Source: CAD feature listing. Evaluate the final solid. Frame: model axes, mm. A direction names the side the tool comes from. Give positions to 0.01 mm unless a question says otherwise; leave off trailing zeros. Order: outer loops, then holes, each group sorted by start corner. A loop starts at its lowest first (then second) coordinate and runs counter-clockwise, first axis right, second up.
from build123d import *

# Parameters (mm, degrees)
SKETCH_2_OUTSIDE_W  = 42.684
SKETCH_2_OUTSIDE_H  = 42.684
CUT_EXTRUDE_1_DEPTH = 30


with BuildPart() as part:
    # Эскиз1 → Повернуть1 (revolve)
    with BuildSketch(Plane.XY, mode=Mode.PRIVATE) as revolve_1_sk:
        Polygon((5, 70), (5, 0), (8.5, 0), (8.5, 60), (12.5, 60), (12.5, 65), (8.5, 65), (8.5, 70), align=None)
    revolve(revolve_1_sk.sketch.rotate(Axis((0, 0, 0), (0, 1, 0)), 90), axis=Axis((0, 0, 0), (0, 1, 0)))

    # Эскиз2 outside → Вырез-Вытянуть1 (cut)
    with BuildSketch(Plane.XZ):
        Rectangle(SKETCH_2_OUTSIDE_W, SKETCH_2_OUTSIDE_H)
        with BuildLine():
            Line((6.5, 3.741657387), (6.5, -3.741657387))
            ThreePointArc((6.5, -3.741657387), (-7.5, 0), (6.5, 3.741657387))
        make_face(mode=Mode.SUBTRACT)
    extrude(amount=-CUT_EXTRUDE_1_DEPTH, mode=Mode.SUBTRACT)


solid = part.part
(1) Section D-D, the plane z = 9.5. Return loops of the section in (x, y).
(2) Access query for faces 1 (the flat face through (-5.3, 0, -0.1)), 2 (the flat face through (6.5, 15, 0)), 3 (the flat face through (8.2, 60, -3)), 4 (the flat face through (8.2, 65, 3)), 5 (the flat face through (4, 70, -4)). Directions: +Z, -Z, +X, -X, +Y, -Y. A direction counts if a zero-diameter tool reaches every point of the face in a straight line with its end or side. Return the directions, or none.
(3) Section B-B, the plane z = 0. Return loops of the section in (x, y).
(4) Pin query (flat end, axial travel): pin 1 Ø10 at (x, y) = (-5, 15.5) entering from +Z; pin 2 Ø6 at (x, y) = (7.5, 9) entering from +Z; pin 3 Ø8 at (x, z) = (9, 3.5) entering from +Y; pin 4 Ø1 at (y, z) = (7.5, -6) entering from +X. Return the tip coordinate at first contact, or that it passes through.
(5) Section C-C, the plane y = 48.5. Return loops of the section in (x, z).
(6) Line query: line 1 along X through (y, z) = (53, 0); line 2 along X through (y, z) = (18.5, 0); line 3 along Y through (x, z) = (-9.25, 7). Output: solid intervals per line, ascending.
(7) Section A-A, the plane x = 0. Return loops of the section in (y, z), plus the area to 3 significant figures.
(8) Draft query along Z for faces 6 (the cylindrical face through (0, 35, 5)), 7 (the cylindrical face through (-8.428, 67.535, 1.107)), 8 (the flat face through (7, 30, 1)). Return one class per face: +Z half, -Z half, draft (parallel to the pull), parting line (faces both ways), or undercut.
Checks:
1. outline: (-8.12, 60) - (8.12, 60) - (8.12, 65) - (-8.12, 65) - close
2. face 1: +Z, -Z, +X, -X, -Y
2. face 2: +Z, -Z, +X, -Y
2. face 3: -Y
2. face 4: +Y
2. face 5: +Z, -Z, +X, -X, +Y
3. outline: (-12.5, 60) - (-8.5, 60) - (-8.5, 30) - (-7.5, 30) - (-7.5, 0) - (-5, 0) - (-5, 70) - (-8.5, 70) - (-8.5, 65) - (-12.5, 65) - close; (5, 0) - (6.5, 0) - (6.5, 30) - (8.5, 30) - (8.5, 60) - (12.5, 60) - (12.5, 65) - (8.5, 65) - (8.5, 70) - (5, 70) - close
4. pin 1: stops at z = 7.5
4. pin 2: stops at z = 6
4. pin 3: stops at y = 70
4. pin 4: stops at x = 5.1
5. outline: circle Ø17 at (0, 0); hole circle Ø10 at (0, 0)
6. line 1: x = -8.5 to -5, 5 to 8.5
6. line 2: x = -7.5 to -5, 5 to 6.5
6. line 3: y = 60 to 65
7. outline: (0, -7.5) - (30, -7.5) - (30, -8.5) - (60, -8.5) - (60, -12.5) - (65, -12.5) - (65, -8.5) - (70, -8.5) - (70, -5) - (0, -5) - close; (0, 5) - (70, 5) - (70, 8.5) - (65, 8.5) - (65, 12.5) - (60, 12.5) - (60, 8.5) - (30, 8.5) - (30, 7.5) - (0, 7.5) - close
7. area: 470 mm2
8. face 6: undercut
8. face 7: parting line
8. face 8: draft
